from build123d import *

# Parameters (mm, degrees)
CYLINDER_R      = 20
CYLINDER_DEPTH  = 3.3
SKETCH_R        = 1.5
POCKET_DEPTH    = 3.301
POCKET001_DEPTH = 5


with BuildPart() as part:
    # Cylinder → Cylinder (new body)
    with BuildSketch(Plane.XY):
        Circle(CYLINDER_R)
    extrude(amount=CYLINDER_DEPTH)

    # Sketch → Pocket (cut, through all)
    with BuildSketch(Plane.XY.offset(3.3)):
        with Locations((0, 15.1)):
            Circle(SKETCH_R)
    extrude(amount=-POCKET_DEPTH, mode=Mode.SUBTRACT)

    # Sketch001 → Pocket001 (cut)
    with BuildSketch(Plane.XY.offset(3.3)):
        Polygon((0, 11), (-9.526279, -5.5), (9.526279, -5.5), align=None)
    extrude(amount=-POCKET001_DEPTH, mode=Mode.SUBTRACT)


solid = part.part
CAD build for the part. Positions are in the model's coordinates, mm. A direction names the side the tool comes from. Coordinates: 2 decimals unless noted, no trailing zeros. Write each loop counter-clockwise with the first axis right and the second up, starting at its lowest first coordinate (ties: lowest second). Pieces come first, ordered by that corner, then holes. Notation, with made-up numbers: M 42,69 L 60,69 A9 cw 60,82 Z; hole C 29.25,-28 d8. An arc over 180 degrees is marked long. Return JSON: item names as keys, results as strings.
Item 1: Slice it at B-B, the plane x = 2. Write the cut outline in (y, z).
Findings below:
{"outline": "M -19.9,0 L -5.5,0 L -5.5,3.3 L -19.9,3.3 Z; M 7.54,0 L 19.9,0 L 19.9,3.3 L 7.54,3.3 Z"}
Item 2: Slice it at C-C, the plane z = 0.7. Write the cut outline in (x, y).
Findings below:
{"outline": "C 0,0 d40; hole M -9.53,-5.5 L 9.53,-5.5 L 0,11 Z; hole C 0,15.1 d3"}
Item 3: Drop flat-ended pins along their axis: pin 1 Ø2.5 at (x, y) = (0, 15.1) entering from -Z; pin 2 Ø1.5 at (x, z) = (6, 2.5) entering from +Y. Give the stop position or say it passes through.
Findings below:
{"pin 1": "passes through", "pin 2": "stops at y = 19.3"}
Item 4: Two-plate mould, pull along Y, no slides. Class faces 3 (the flat face through (4, 5, 0)), 4 (the flat face through (0, -5.5, 2)), 5 (the flat face through (4.83, 2.635, 1.673)), 6 (the cylindrical face through (-4.336, -19.524, 1.627)): +Y half, -Y half, draft (parallel to the pull), parting line (faces both ways), or undercut.
Findings below:
{"face 3": "draft", "face 4": "undercut", "face 5": "undercut", "face 6": "parting line"}
Item 5: Which spindle directions (+Z, -Z, +X, -X, +Y, -Y) get a long thin tool onto all of the face, cutting with end or side? Do faces 1 (the flat face through (-4.696, 2.865, 1.673)), 2 (the flat face through (4, 5, 3.3)). Say none if no direction does.
Findings below:
{"face 1": "+Z, -Z", "face 2": "+Z, +X, -X, +Y, -Y"}
Item 6: Slice it at A-A, the plane y = -3. Write the cut outline in (x, z), and give its area (3 significant figures).
Findings below:
{"outline": "M -19.77,0 L -8.08,0 L -8.08,3.3 L -19.77,3.3 Z; M 8.08,0 L 19.77,0 L 19.77,3.3 L 8.08,3.3 Z", "area": "77.2 mm2"}
Item 7: Slice it at D-D, the plane y = -12. Write the cut outline in (x, z).
Findings below:
{"outline": "M -16,0 L 16,0 L 16,3.3 L -16,3.3 Z"}
Item 8: Probe line 1 (Y direction, x = -1, z = 1.95); line 2 (Y direction, x = 8, z = 2.4); line 3 (Y direction, x = 6, z = 2.7). List the from-to ranges inside material, lowest first. Write a range as from..to.
Findings below:
{"line 1": "y = -19.97..-5.5, 9.27..13.98, 16.22..19.97", "line 2": "y = -18.33..-5.5, -2.86..18.33", "line 3": "y = -19.08..-5.5, 0.61..19.08"}
